Read the model definition and answer for the solid it produces. Units are mm, in the model's axes. A direction names the side the tool comes from. Coordinates: 2 decimals unless noted, no trailing zeros. Loops run counter-clockwise (first coordinate to the right, second up) from the corner with the lowest first, then second, coordinate; pieces in that order, holes last. Notation, with made-up numbers: M 40,-18.75 L 66,-18.75 A26 cw 66,11.25 Z; hole C 89,-34 d10. An arc over 180 degrees is marked long. Use one line per item in the form item = value. Start each with the question number.
1. The part is cut by section B-B (y = 19.5). Give the vertices of the cut face in (x, z) (3 decimals).
2. Find the intervals of material crossed by probe 1 along Z at (x, y) = (1, 21.3); probe 2 along X at (y, z) = (-0.5, 26.5); probe 3 along Z at (x, y) = (-44, -4), in increasing order. Write a range as [from, to].
3. For a pull along X with two mould halves and no side action, classify faces 6 (the flat face through (-100, 0, 1)), 7 (the flat face through (99, -22.5, 0)), 8 (the flat face through (37.5, -14, 34)), 9 (the flat face through (87, -13, 35)) as released by +X, released by -X, zero draft, split by the parting line, or undercut.
4. Flat-ended cylindrical pins translate along their axes: pin 1 (1.6 mm diameter, centred on x = 1, z = -27.49, fed in from -Y); pin 2 (3 mm diameter, centred on x = 88, y = -17.5, fed in from +Z); pin 3 (6 mm diameter, centred on x = 6.5, y = -10.5, fed in from +Z). Find the tip coordinate at first contact, or state that the pin passes through.
5. The part is cut by section A-A (x = -31). Give the vertices of the cut face in (y, z).
6. A tool of negligible diameter and unlimited length cuts with its end or side. For faces 1 (the flat face through (-1, -5, 34)), 2 (the flat face through (-95, -2, -1)), 3 (the flat face through (-12.75, 20, 24)), 4 (the flat face through (87, -17, 32.5)), 5 (the flat face through (-1, 22.5, -1)), from which of +Z, -Z, +X, -X, +Y, -Y can it reach the whole face along a straight path? Write none if from no direction.
7. The part is cut by section D-D (y = -18.5). Give the vertices of the cut face in (x, z), plus the area to 3 significant figures.
8. The part is cut by section C-C (z = -30.5). Give the vertices of the cut face in (x, y).
from build123d import *

# Parameters (mm, degrees)
SKETCH1_W                 = 200
SKETCH1_H                 = 75
BOSS_EXTRUDE1_DEPTH       = 22.5
SHELL1_T                  = -5
SKETCH2_W                 = 23
SKETCH2_H                 = 12.75
CUT_EXTRUDE1_DEPTH        = 116.893269865
SKETCH4_W                 = 190
SKETCH4_H                 = 40
BOSS_EXTRUDE2_DEPTH       = 2.5
SKETCH5_W                 = 6
SKETCH5_H                 = 8.5
SKETCH5_W_2               = 5
SKETCH5_H_2               = 7.5
CUT_EXTRUDE2_DEPTH        = 5
F_1_0MM_DOWEL_HOLE1_D     = 15
F_1_0MM_DOWEL_HOLE1_DEPTH = 5
F_1_0MM_DOWEL_HOLE1_TIP   = 4.506454643
SKETCH9_W                 = 75
SKETCH9_H                 = 17.5
CUT_EXTRUDE3_DEPTH        = 7.5
SKETCH10_W                = 2.5
SKETCH10_H                = 7.5
CUT_EXTRUDE4_DEPTH        = 5
F_1_0MM_DOWEL_HOLE2_D     = 1.25
F_1_0MM_DOWEL_HOLE2_DEPTH = 5
F_1_0MM_DOWEL_HOLE2_TIP   = 0.375537887


with BuildPart() as part:
    # Sketch1 → Boss-Extrude1 (new, symmetric)
    with BuildSketch(Plane(origin=(0, 0, 0), x_dir=(1, 0, 0), z_dir=(0, 1, 0))):
        Rectangle(SKETCH1_W, SKETCH1_H)
    extrude(amount=BOSS_EXTRUDE1_DEPTH, both=True)

    # Shell1
    shell1_openings = [part.faces().sort_by_distance(p)[0] for p in [
        (0, -22.5, 0),
    ]]
    offset(amount=SHELL1_T, openings=shell1_openings, kind=Kind.INTERSECTION)

    # Sketch2 → Cut-Extrude1 (cut, through all)
    with BuildSketch(Plane(origin=(0, 22.5, 0), x_dir=(1, 0, 0), z_dir=(0, 1, 0))):
        with Locations((0, -23.625)):
            Rectangle(SKETCH2_W, SKETCH2_H)
    extrude(amount=-CUT_EXTRUDE1_DEPTH, mode=Mode.SUBTRACT)

    # Sketch4 → Boss-Extrude2 (add)
    with BuildSketch(Plane(origin=(0, 0, 32.5), x_dir=(-1, 0, 0), z_dir=(0, 0, -1))):
        with Locations((0, -2.5)):
            Rectangle(SKETCH4_W, SKETCH4_H)
    extrude(amount=BOSS_EXTRUDE2_DEPTH)

    # Sketch5 → Cut-Extrude2 (cut)
    # profile 1 of 8: a face of its own
    with BuildSketch(Plane.XY.offset(37.5)):
        with Locations((-87.5, -2.75)):
            Rectangle(SKETCH5_W, SKETCH5_H)
        with Locations((-87.5, -2.75)):
            Rectangle(SKETCH5_W_2, SKETCH5_H_2, mode=Mode.SUBTRACT)
    # profile 2 of 8: a face of its own
    with BuildSketch(Plane.XY.offset(37.5)):
        with Locations((-87.5, -2.75)):
            Rectangle(SKETCH5_W_2, SKETCH5_H_2)
    # profile 3 of 8: a face of its own
    with BuildSketch(Plane.XY.offset(37.5)):
        with Locations((-87.5, -17.25)):
            Rectangle(SKETCH5_W, SKETCH5_H)
        with Locations((-87.5, -17.25)):
            Rectangle(SKETCH5_W_2, SKETCH5_H_2, mode=Mode.SUBTRACT)
    # profile 4 of 8: a face of its own
    with BuildSketch(Plane.XY.offset(37.5)):
        with Locations((-87.5, -17.25)):
            Rectangle(SKETCH5_W_2, SKETCH5_H_2)
    # profile 5 of 8: a face of its own
    with BuildSketch(Plane.XY.offset(37.5)):
        with Locations((87.5, -2.75)):
            Rectangle(SKETCH5_W, SKETCH5_H)
        with Locations((87.5, -2.75)):
            Rectangle(SKETCH5_W_2, SKETCH5_H_2, mode=Mode.SUBTRACT)
    # profile 6 of 8: a face of its own
    with BuildSketch(Plane.XY.offset(37.5)):
        with Locations((87.5, -2.75)):
            Rectangle(SKETCH5_W_2, SKETCH5_H_2)
    # profile 7 of 8: a face of its own
    with BuildSketch(Plane.XY.offset(37.5)):
        with Locations((87.5, -17.25)):
            Rectangle(SKETCH5_W, SKETCH5_H)
        with Locations((87.5, -17.25)):
            Rectangle(SKETCH5_W_2, SKETCH5_H_2, mode=Mode.SUBTRACT)
    # profile 8 of 8: a face of its own
    with BuildSketch(Plane.XY.offset(37.5)):
        with Locations((87.5, -17.25)):
            Rectangle(SKETCH5_W_2, SKETCH5_H_2)
    extrude(amount=-CUT_EXTRUDE2_DEPTH, mode=Mode.SUBTRACT)

    # Ø1.0mm Dowel Hole1
    with Locations(Plane(origin=(0, 0, -37.5), x_dir=(-1, 0, 0), z_dir=(0, 0, -1))):
        with Locations((0, -22.5)):
            Hole(F_1_0MM_DOWEL_HOLE1_D / 2, depth=F_1_0MM_DOWEL_HOLE1_DEPTH)
            with Locations((0, 0, -(F_1_0MM_DOWEL_HOLE1_DEPTH + F_1_0MM_DOWEL_HOLE1_TIP / 2))):  # 118° drill point
                Cone(0, F_1_0MM_DOWEL_HOLE1_D / 2, F_1_0MM_DOWEL_HOLE1_TIP, mode=Mode.SUBTRACT)

    # Sketch9 → Cut-Extrude3 (cut)
    with BuildSketch(Plane.XY.offset(37.5)):
        with Locations((0, -13.75)):
            Rectangle(SKETCH9_W, SKETCH9_H)
    extrude(amount=-CUT_EXTRUDE3_DEPTH, mode=Mode.SUBTRACT)

    # Sketch10 → Cut-Extrude4 (cut)
    with BuildSketch(Plane(origin=(0, 22.5, 0), x_dir=(1, 0, 0), z_dir=(0, 1, 0))):
        with Locations((-11.5, -23.625)):
            Rectangle(SKETCH10_W, SKETCH10_H)
    extrude(amount=-CUT_EXTRUDE4_DEPTH, mode=Mode.SUBTRACT)

    # Ø1.0mm Dowel Hole2
    with Locations(Plane(origin=(0, 22.5, 0), x_dir=(1, 0, 0), z_dir=(0, 1, 0))):
        with Locations((-0.999952175, 27.490220049), (1.000000001, 27.490219113), (-44.767078272, 1.066584153), (-43.767078272, 2.79863496), (43.767078272, 2.79863496), (44.76705517, 1.066626038)):
            Hole(F_1_0MM_DOWEL_HOLE2_D / 2, depth=F_1_0MM_DOWEL_HOLE2_DEPTH)
            with Locations((0, 0, -(F_1_0MM_DOWEL_HOLE2_DEPTH + F_1_0MM_DOWEL_HOLE2_TIP / 2))):  # 118° drill point
                Cone(0, F_1_0MM_DOWEL_HOLE2_D / 2, F_1_0MM_DOWEL_HOLE2_TIP, mode=Mode.SUBTRACT)


solid = part.part
Computed values:
q1.outline = M -100,-37.5 L 100,-37.5 L 100,37.5 L -100,37.5 Z; hole C -44.767,-1.067 d1.25; hole C -43.767,-2.799 d1.25; hole M -12.75,19.875 L -11.5,19.875 L -11.5,17.25 L 11.5,17.25 L 11.5,30 L -11.5,30 L -11.5,27.375 L -12.75,27.375 Z; hole C -1,-27.49 d1.25; hole C 1,-27.49 d1.25; hole C 43.767,-2.799 d1.25; hole C 44.767,-1.067 d1.25
q2.probe_1 = [-37.5, -28.12], [-26.87, 17.25], [30, 37.5]
q2.probe_2 = [-100, -95], [95, 100]
q2.probe_3 = [-37.5, -32.5], [30, 37.5]
q3.face_6 = released by -X
q3.face_7 = zero draft
q3.face_8 = undercut
q3.face_9 = undercut
q4.pin_1 = 17.5
q4.pin_2 = 32.5
q4.pin_3 = -32.5
q5.outline = M -22.5,-37.5 L 22.5,-37.5 L 22.5,37.5 L -5,37.5 L -5,30 L 17.5,30 L 17.5,-32.5 L -22.5,-32.5 Z
q6.face_1 = +Z, -Y
q6.face_2 = -Y
q6.face_3 = +Y, -Y
q6.face_4 = +Z
q6.face_5 = +Z, -Z, +X, -X, +Y
q7.outline = M -100,-37.5 L -6.34,-37.5 L -6.34,-32.5 L -95,-32.5 L -95,30 L -37.5,30 L -37.5,37.5 L -84.5,37.5 L -84.5,32.5 L -90.5,32.5 L -90.5,37.5 L -100,37.5 Z; M 6.34,-37.5 L 100,-37.5 L 100,37.5 L 90.5,37.5 L 90.5,32.5 L 84.5,32.5 L 84.5,37.5 L 37.5,37.5 L 37.5,30 L 95,30 L 95,-32.5 L 6.34,-32.5 Z
q7.area = 2,440 mm²
q8.outline = M -100,-22.5 L -95,-22.5 L -95,17.5 L 95,17.5 L 95,-22.5 L 100,-22.5 L 100,22.5 L -100,22.5 Z
